Autodesk Inventor part; units mm, degrees
ref_plane "YZ Plane" through (0, 0, 0) normal (1, 0, 0) x (0, 1, 0)
ref_plane "XZ Plane" through (0, 0, 0) normal (0, 1, 0) x (-1, 0, 0)
ref_plane "XY Plane" through (0, 0, 0) normal (0, 0, 1) x (1, 0, 0)
sketch "Sketch1" plane through (0, 0, 0) normal (0, 0, 1) x (1, 0, 0)
  line L0 (0, 85.0385) -> (0, 91.0385)
  line L1 (-9, 91.0385) -> (-10, 91.0385)
  line L2 (0, 61.1) -> (0, 78.9)
  line L3 (0, 91.0385) -> (0, 96.0385)
  line L4 (-10, 91.0385) -> (-11, 91.0385)
  line L5 (-9, 91.0385) -> (-9, 85.0385)
  line L6 (-11, 91.0385) -> (-8.1132, 96.0385)
  line L7 (0, 96.0385) -> (0, 109.0385)
  line L8 (0, 96.0385) -> (0, 102.5385) construction
  line L9 (0, 102.5385) -> (-10.5, 102.5385) construction
  line L10 (-11, 114.0385) -> (-8.1132, 109.0385)
  line L11 (0, 114.0385) -> (-8, 114.0385)
  line L12 (-10, 114.0385) -> (-11, 114.0385)
  line L13 (0, 114.0385) -> (-10, 114.0385)
  line L14 (0, 109.0385) -> (0, 114.0385)
  line L15 (-8.1132, 96.0385) -> (-8.1132, 109.0385)
  line L16 (0, 0) -> (0, 114.0385)
  line L17 (0, 85.0385) -> (0, 0)
  line L18 (14, 0) -> (-14, 0)
  line L19 (0, 78.9) -> (-9, 79.0832)
  line L20 (-12, 79.0832) -> (12, 79.0832)
  line L21 (-9, 79.0832) -> (-9, 85.0385)
  point P0 (-8, 264.0385)
  point P1 (-9, 241.0385)
  point P2 (0, 79.0832)
  dimension "d0" = 6
  dimension "d1" = 10
  dimension "d2" = 5
  dimension "d3" = 9
  dimension "d4" = 13
revolve "Revolution1" add sketch "Sketch1" angle 360 about axis through (0, 0, 0) along (0, 1, 0) contours L16 L20 L21 L5 L1 L4 L6 L15 L10 L12 L13 L11 L14 L7 L3 L0
sketch "Sketch2" plane through (0, 0, 0) normal (0, 0, 1) x (1, 0, 0)
  line L0 (8.1132, 109.0385) -> (11, 114.0385) construction
  line L1 (8.1132, 109.0385) -> (8.1132, 112.5385) construction
  line L2 (8.1132, 112.5385) -> (9.0002, 112.5385) construction
  line L3 (9.0002, 114.0385) -> (9.8662, 114.0385)
  line L4 (11, 114.0385) -> (-11, 114.0385)
  line L5 (9.8662, 114.0385) -> (9.0002, 112.5385)
  line L6 (8.1132, 109.0385) -> (-8.1132, 109.0385)
  line L7 (9.0002, 112.5385) -> (0, 112.5385)
  line L8 (9.0002, 114.0385) -> (0, 114.0385)
  line L9 (0, 109.0385) -> (0, 117.7347)
  point P0 (0, 0)
  point P1 (0, 112.5385)
  dimension "d6" = 3.5
  dimension "d7" = 0.887
  dimension "d8" = 1.5
  dimension "d9" = 0.866
revolve "Revolution2" cut sketch "Sketch2" angle 360 about axis through (0, 109.0385, 0) along (0, 1, 0)
fillet "Fillet1" radius 0.3 1 edges at (11, 114.0385, 0)
fillet "Fillet2" radius 0.3 1 edges at (11, 91.0385, 0)
sketch "Sketch3" plane through (0, 79.0832, 0) normal (0, -1, 0) x (1, 0, 0)
  circle A0 centre (0, 0) radius 5
  dimension "d13" = 10
extrude "Extrusion1" cut sketch "Sketch3" against normal blind 15
properties part number "emitter"
Part model, mm, in its own coordinate system. A direction names the side the tool comes from. Round coordinates to 2 decimals unless told otherwise and drop trailing zeros. Order: outer loops, then holes, each group sorted by start corner. A loop starts at its lowest first (then second) coordinate and runs counter-clockwise, first axis right, second up. Notation, with made-up numbers: M 54,19.5 L 67,19.5 A24 cw 67,56.5 Z; hole C 87,36.25 d3. An arc over 180 degrees is marked long. Put each result on its own line as item: value. Start each with the question number.
1. Slice it at D-D on y = 103. List the corners of the cut face in (x, z).
2. Slice it at C-C on y = 81. List the corners of the cut face in (x, z), then the cut area to 3 significant figures.
3. Tool access for faces 1 (the face through (-7.739, 102.63, 2.437)), 2 (the face through (-4, 79.083, -4)), 3 (the face through (-1.08, 86.48, -4.88)): list every direction of +Z, -Z, +X, -X, +Y, -Y with a clear straight run to the whole face (end or side of a thin tool).
4. Slice it at B-B on x = 0. List the corners of the cut face in (y, z), then the cut area to 3 significant figures.
5. Slice it at A-A on z = 0. List the corners of the cut face in (x, y).
6. Drill centre lines: probe 1 along Z at (x, y) = (0, 88.5); probe 2 along Y at (x, z) = (3.75, -2); probe 3 along Y at (x, z) = (-5, 5.25). Where is each one in solid material? Low to high. Write a range as [from, to].
7. Drop flat-ended pins along their axis: pin 1 (2 mm diameter, centred on x = -6.5, y = 110.5, fed in from +Z); pin 2 (6 mm diameter, centred on x = 0, z = 0, fed in from +Y); pin 3 (2 mm diameter, centred on y = 101, z = -4.5, fed in from +X). Give the stop position or say it passes through.
8. Two-plate mould, pull along Z, no slides. Class faces 4 (the face through (-9.3, 114.038, -3.8)), 5 (the face through (0, 112.538, 0)), 6 (the face through (-7.895, 95.754, -2.486)): +Z half, -Z half, draft (parallel to the pull), parting line (faces both ways), or undercut.
Findings:
1. outline: C 0,0 d16.23
2. outline: C 0,0 d18; hole C 0,0 d10
2. area: 176 mm2
3. face 1: none
3. face 2: +Z, -Z, +X, -X, -Y
3. face 3: -Y
4. outline: M 79.08,-9 L 91.04,-9 L 91.04,-10.48 A0.3 ccw 91.49,-10.74 L 96.04,-8.11 L 109.04,-8.11 L 113.59,-10.74 A0.3 ccw 114.04,-10.48 L 114.04,-9.87 L 112.54,-9 L 112.54,9 L 114.04,9.87 L 114.04,10.48 A0.3 ccw 113.59,10.74 L 109.04,8.11 L 96.04,8.11 L 91.49,10.74 A0.3 ccw 91.04,10.48 L 91.04,9 L 79.08,9 L 79.08,5 L 94.08,5 L 94.08,-5 L 79.08,-5 Z
4. area: 439 mm2
5. outline: M -10.74,91.49 A0.3 ccw -10.48,91.04 L -9,91.04 L -9,79.08 L -5,79.08 L -5,94.08 L 5,94.08 L 5,79.08 L 9,79.08 L 9,91.04 L 10.48,91.04 A0.3 ccw 10.74,91.49 L 8.11,96.04 L 8.11,109.04 L 10.74,113.59 A0.3 ccw 10.48,114.04 L 9.87,114.04 L 9,112.54 L -9,112.54 L -9.87,114.04 L -10.48,114.04 A0.3 ccw -10.74,113.59 L -8.11,109.04 L -8.11,96.04 Z
6. probe 1: [-9, -5], [5, 9]
6. probe 2: [94.08, 112.54]
6. probe 3: [79.08, 112.54]
7. pin 1: z = 7.36
7. pin 2: y = 112.54
7. pin 3: x = 7.32
8. face 4: draft
8. face 5: undercut
8. face 6: parting line
